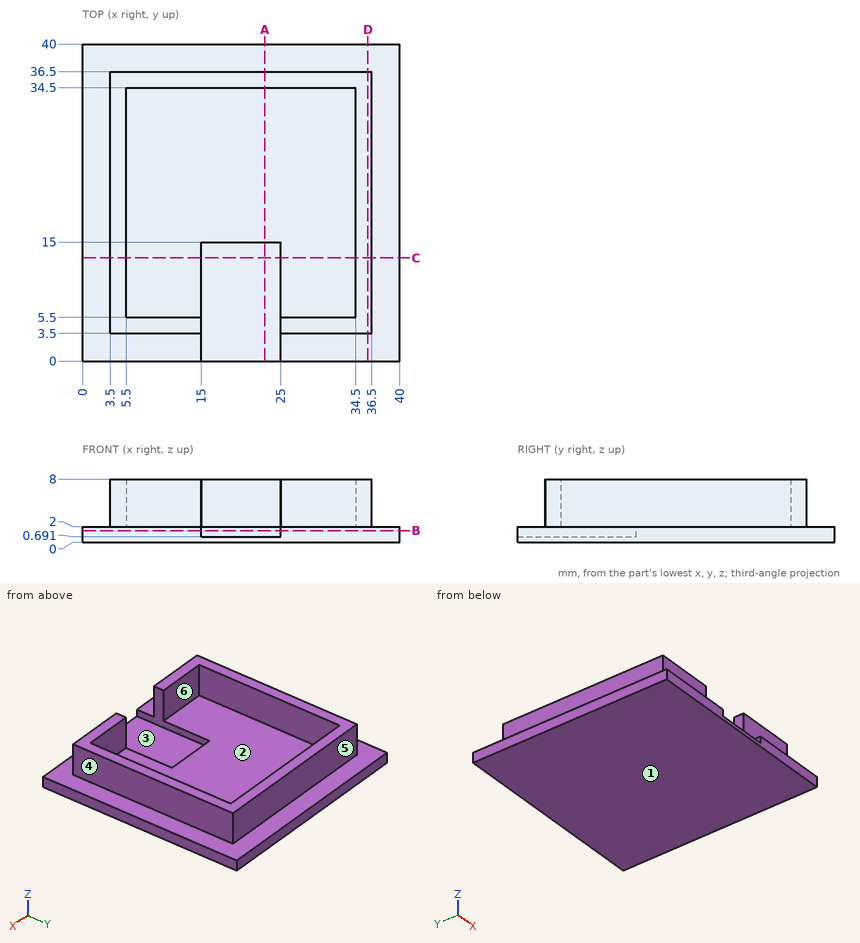
Part print with two shaded views. Sizes in mm from the minimum x, y, z corner. A direction names the side the tool comes from. Coordinates: 2 decimals unless noted, no trailing zeros. Write each loop counter-clockwise with the first axis right and the second up, starting at its lowest first coordinate (ties: lowest second). Pieces come first, ordered by that corner, then holes. Notation, with made-up numbers: (12.25, 50.25) - (32.25, 50.25) arc R19 cw to (32.25, 68.25) - close; hole circle Ø1 at (10, 16). An arc over 180 degrees is marked (long way). Put each result on its own line as item: value.
1. Band-saw the part on D-D (x = 36). Write the cut outline in (y, z), then the cut area to 3 significant figures.
Final values:
outline: (0, 0) - (40, 0) - (40, 2) - (36.5, 2) - (36.5, 8) - (3.5, 8) - (3.5, 2) - (0, 2) - close
area: 278 mm²
2. Probe line 1 along X through (y, z) = (28, 3.25); line 2 along Y through (x, z) = (21, 6.25). List the from-to ranges inside material, lowest first. Write a range as [from, to].
Final values:
line 1: x = [3.5, 5.5], [34.5, 36.5]
line 2: y = [34.5, 36.5]
3. Band-saw the part on C-C (y = 13). Write the cut outline in (x, z).
Final values:
outline: (0, 0) - (40, 0) - (40, 2) - (36.5, 2) - (36.5, 8) - (34.5, 8) - (34.5, 2) - (25, 2) - (25, 0.69) - (15, 0.69) - (15, 2) - (5.5, 2) - (5.5, 8) - (3.5, 8) - (3.5, 2) - (0, 2) - close
4. Flat gauge pins, fed straight in: pin 1 Ø1 at (y, z) = (27.5, 6.5) entering from -X; pin 2 Ø2 at (y, z) = (5, 4) entering from +X; pin 3 Ø1 at (x, z) = (30.5, 4) entering from +Y; pin 4 Ø8 at (x, y) = (13.5, 21) entering from -Z. Where does each tip first touch, or does it go through?
Final values:
pin 1: stops at x = 3.5
pin 2: stops at x = 36.5
pin 3: stops at y = 36.5
pin 4: stops at z = 0
5. Band-saw the part on A-A (x = 23). Write the cut outline in (y, z).
Final values:
outline: (0, 0) - (40, 0) - (40, 2) - (36.5, 2) - (36.5, 8) - (34.5, 8) - (34.5, 2) - (15, 2) - (15, 0.69) - (0, 0.69) - close
6. Two-plate mould, pull along X, no slides. Class the marked faces 3, 4, 5 and 6: +X half, -X half, draft (parallel to the pull), parting line (faces both ways), or undercut.
Final values:
face 3: undercut
face 4: +X half
face 5: draft
face 6: undercut
7. Band-saw the part on B-B (z = 1.5). Write the cut outline in (x, y).
Final values:
outline: (0, 0) - (15, 0) - (15, 15) - (25, 15) - (25, 0) - (40, 0) - (40, 40) - (0, 40) - close
8. 3-axis set-ups, long thin cutter, end or side, ignore diameter. For the marked faces 1 and 2: which of +Z, -Z, +X, -X, +Y, -Y reach the whole face in a straight line?
Final values:
face 1: -Z, +X, -X, +Y, -Y
face 2: +Z
